from build123d import *

# Parameters (mm, degrees)
F0_R            = 30.5
F0_R_2          = 9.5
F1_DEPTH        = 2
F2_R            = 32
F2_R_2          = 30.5
F3_DEPTH        = 17
F4_R            = 3
F5_DEPTH        = 17
F5_COPIES_COUNT = 3
F6_R            = 31.25
F7_DEPTH        = 2
F8_W            = 5
F8_H            = 4
F9_DEPTH        = 43.1
F10_R           = 5
F11_DEPTH       = 10
F13_DEPTH       = 25


# Not quite as in the source:
# - a pattern or mirror of a feature is missing from the dataset's text; its kind, count and spacing are read off the source's solid


with BuildPart() as f1:
    # F0 (on Right) → F1 (new body)
    with BuildSketch(Plane.YZ):
        Circle(F0_R)
        Circle(F0_R_2, mode=Mode.SUBTRACT)
    extrude(amount=F1_DEPTH)

    # F2 (on face) → F3 (join)
    with BuildSketch(Plane(origin=(0, 0, 0), x_dir=(0, -1, 0), z_dir=(-1, 0, 0))):
        Circle(F2_R)
        Circle(F2_R_2, mode=Mode.SUBTRACT)
    extrude(amount=-F3_DEPTH)

    # F4 (on face) → F5 (join)
    with BuildSketch(Plane.YZ.offset(17)):
        with BuildLine():
            ThreePointArc((-6.5, 42), (0, 35.5), (6.5, 42))
            ThreePointArc((6.5, 42), (0, 48.5), (-6.5, 42))
        make_face()
        with Locations((0, 42)):
            Circle(F4_R, mode=Mode.SUBTRACT)
        with BuildLine():
            Line((7, 31.224989992), (6.5, 42))
            ThreePointArc((6.5, 42), (0, 35.5), (-6.5, 42))
            Line((-6.5, 42), (-7, 31.224989992))
            ThreePointArc((-7, 31.224989992), (0, 32), (7, 31.224989992))
        make_face()
    f5 = extrude(amount=-F5_DEPTH)

    # F5_copies: F5 ×3 about axis
    f5_copies_axis = Axis((0, 0, 0), (1, 0, 0))
    for i in range(1, F5_COPIES_COUNT):
        add(f5.rotate(f5_copies_axis, i * 360 / F5_COPIES_COUNT))

    # F6 (on face) → F7 (cut)
    with BuildSketch(Plane.YZ.offset(17)):
        Circle(F6_R)
    extrude(amount=-F7_DEPTH, mode=Mode.SUBTRACT)

    # F8 (on Front) → F9 (cut)
    with BuildSketch(Plane.XZ):
        with Locations((9.5, 2)):
            Rectangle(F8_W, F8_H)
    extrude(amount=-F9_DEPTH, mode=Mode.SUBTRACT)

    # F10 (on face) → F11 (cut)
    with BuildSketch(Plane(origin=(0, 0, 0), x_dir=(0, -1, 0), z_dir=(-1, 0, 0))):
        with Locations((-36.3730669589, -21)):
            Circle(F10_R)
        with Locations((0, 42)):
            Circle(F10_R)
        with Locations((36.3730669589, -21)):
            Circle(F10_R)
    extrude(amount=-F11_DEPTH, mode=Mode.SUBTRACT)

    # F12 (on face) → F13 (cut)
    with BuildSketch(Plane(origin=(0, 0, 0), x_dir=(0, -1, 0), z_dir=(-1, 0, 0))):
        with BuildLine():
            Line((-12.5, 0), (-20, 0))
            ThreePointArc((-20, 0), (-14.1421356237, -14.1421356237), (0, -20))
            Line((0, -20), (0, -12.5))
            ThreePointArc((0, -12.5), (8.8388347648, -8.8388347648), (12.5, 0))
            Line((12.5, 0), (20, 0))
            ThreePointArc((20, 0), (14.1421356237, 14.1421356237), (0, 20))
            Line((0, 20), (0, 12.5))
            ThreePointArc((0, 12.5), (-8.8388347648, 8.8388347648), (-12.5, 0))
        make_face()
    extrude(amount=-F13_DEPTH, mode=Mode.SUBTRACT)


solid = f1.part
Here's how the part is built. I have some questions about the finished solid (model axes, mm). A direction names the side the tool comes from. Coordinates: 2 decimals unless noted, no trailing zeros. Write each loop counter-clockwise with the first axis right and the second up, starting at its lowest first coordinate (ties: lowest second). Pieces come first, ordered by that corner, then holes. Notation, with made-up numbers: (34.5, 68) - (64.5, 68) arc R16 ccw to (64.5, 91) - close; hole circle Ø2 at (34, 50.5). An arc over 180 degrees is marked (long way). Use one line per item in the form item = value.
1) Suppose I cut it at C-C, the plane z = 38. Write out the boundary of the cut face in (x, y), plus the area to 3 significant figures.
Solved:
outline = (0, -6.69) - (17, -6.69) - (17, 6.69) - (0, 6.69) - (0, 3) - (10, 3) - (10, -3) - (0, -3) - close
area = 167 mm2
2) Suppose I cut it at D-D, the plane z = 29.5. Write out the boundary of the cut face in (x, y), plus the area to 3 significant figures.
Solved:
outline = (0, -12.4) - (17, -12.4) - (17, -10.31) - (15, -10.31) - (15, -7.75) - (2, -7.75) - (2, 7.75) - (15, 7.75) - (15, 10.31) - (17, 10.31) - (17, 12.4) - (0, 12.4) - close
area = 179 mm2
3) Thinking about a two-plate mould opening in Y: for faces 5 (the cylindrical face through (0.986, 8.741, 8.935)), 6 (the flat face through (8.619, -6.746, 36.688)), 7 (the flat face through (8.619, 6.754, 36.537)), which applies, released by +Y, released by -Y, zero draft, split by the parting line, or undercut?
Solved:
face_5 = undercut
face_6 = released by -Y
face_7 = released by +Y
4) On a 3-axis mill with a long thin cutter (end or side, diameter ignored), from which of +Z, -Z, +X, -X, +Y, -Y can I reach the whole of each face in a straight line? I mean faces 1 (the cylindrical face through (16.01, -31.22, 1.37)), 2 (the flat face through (10, 0.1, 38.7)), 3 (the flat face through (8.62, -35.02, -12.42)), 4 (the flat face through (1, 16, 0)). Say none if no direction works.
Solved:
face_1 = +X
face_2 = -X
face_3 = +X, -X, -Y
face_4 = +X, -X
5) Suppose I cut it at B-B, the plane y = 14. Write out the boundary of the cut face in (x, z).
Solved:
outline = (0, -28.77) - (17, -28.77) - (17, -27.94) - (15, -27.94) - (15, -27.1) - (2, -27.1) - (2, -14.28) - (0, -14.28) - close; (0, 0) - (2, 0) - (2, 27.1) - (15, 27.1) - (15, 27.94) - (17, 27.94) - (17, 28.77) - (0, 28.77) - close
6) I'm going to push flat-ended pins straight in: P1, Ø2, axis at x = 1.5, z = 15.5, coming from the -Y side; P2, Ø1, axis at x = 14.5, z = 27.5, coming from the +Y side; P3, Ø3, axis at y = 16, z = 21.5, coming from the +X side. Where does each tip first touch, or does it pass through?
Solved:
P1 = -28.53
P2 = 17.18
P3 = 2
7) I need wall thicknesses on line 1 (Z direction, x = 8.25, y = 0); line 2 (X direction, y = 31, z = 2); line 3 (X direction, y = 23, z = -18). Which ranges of each line are inside material? Lowest first, please.
Solved:
line_1 = -32 to -30.5, 30.5 to 37, 47 to 48.5
line_2 = 0 to 7, 12 to 15
line_3 = 0 to 2
8) Suppose I cut it at A-A, the plane z = 19. Write out the boundary of the cut face in (x, y) (3 decimals), plus the area to 3 significant figures.
Solved:
outline = (0, -25.749) - (17, -25.749) - (17, -24.811) - (15, -24.811) - (15, -23.859) - (2, -23.859) - (2, -6.245) - (0, -6.245) - close; (0, 0) - (2, 0) - (2, 23.859) - (15, 23.859) - (15, 24.811) - (17, 24.811) - (17, 25.749) - (0, 25.749) - close
area = 143 mm2
